from build123d import *

# Parameters (mm, degrees)
SKETCH_1_R          = 25.5
EXTRUDE_1_DEPTH     = 13
SKETCH_2_R          = 23.5
CUT_EXTRUDE_1_DEPTH = 11
SKETCH_3_R          = 22
CUT_EXTRUDE_2_DEPTH = 2
EXTRUDE_START       = -3
SKETCH_4_R          = 35.5
SKETCH_4_R_2        = 25.5
EXTRUDE_2_DEPTH     = 3
SKETCH_5_R          = 1.575
CUT_EXTRUDE_3_DEPTH = 52.860389509


with BuildPart() as part:
    # 草图1 → 凸台-拉伸1 (new body)
    with BuildSketch(Plane.XY):
        with Locations(Location((0, 0, 0), (0, 0, 180))):
            Circle(SKETCH_1_R)
    extrude(amount=EXTRUDE_1_DEPTH)

    # 草图2 → 切除-拉伸1 (cut)
    with BuildSketch(Plane(origin=(0, 0, 0), x_dir=(-1, 0, 0), z_dir=(0, 0, -1))):
        Circle(SKETCH_2_R)
    extrude(amount=-CUT_EXTRUDE_1_DEPTH, mode=Mode.SUBTRACT)

    # 草图3 → 切除-拉伸2 (cut)
    with BuildSketch(Plane.XY.offset(13)):
        Circle(SKETCH_3_R)
    extrude(amount=-CUT_EXTRUDE_2_DEPTH, mode=Mode.SUBTRACT)

    # 草图4 → 凸台-拉伸2 (add)
    with BuildSketch(Plane.XY.offset(13).offset(EXTRUDE_START)):
        Circle(SKETCH_4_R)
        with Locations(Location((0, 0, 0), (0, 0, 180))):
            Circle(SKETCH_4_R_2, mode=Mode.SUBTRACT)
    extrude(amount=EXTRUDE_2_DEPTH)

    # 草图5 → 切除-拉伸3 (cut, through all)
    with BuildSketch(Plane.XY.offset(13)):
        with Locations((0, 30.5)):
            Circle(SKETCH_5_R)
        with Locations((30.5, 0)):
            Circle(SKETCH_5_R)
        with Locations((0, -30.5)):
            Circle(SKETCH_5_R)
        with Locations((-30.5, 0)):
            Circle(SKETCH_5_R)
    extrude(amount=-CUT_EXTRUDE_3_DEPTH, mode=Mode.SUBTRACT)


solid = part.part
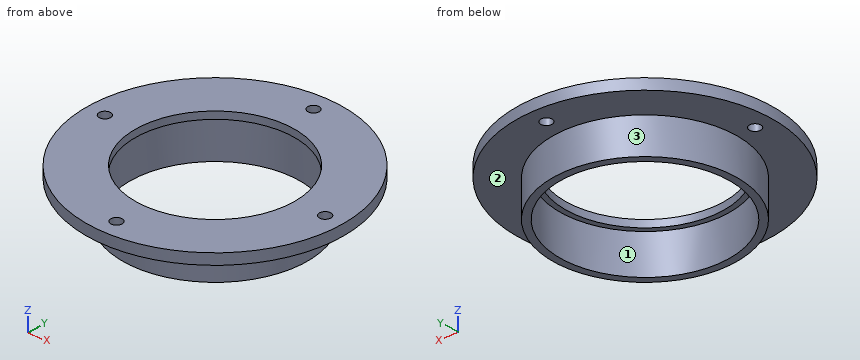
Work out the finished part from the listing and answer in its coordinate system (mm). Face numbers are marked on the shaded views. Round coordinates to 2 decimals unless told otherwise and drop trailing zeros. Write each loop counter-clockwise with the first axis right and the second up, starting at its lowest first coordinate (ties: lowest second). Pieces come first, ordered by that corner, then holes. Notation, with made-up numbers: (31.5, 49.25) - (45.5, 49.25) arc R18 cw to (45.5, 71.25) - close; hole circle Ø10 at (-20, 37.5). An arc over 180 degrees is marked (long way). Answer in a Markdown table with one row per item. Add a question column.
1. Given pin 1 (5 mm diameter, centred on x = 0, y = -30.5, fed in from +Z); pin 2 (1.9 mm diameter, centred on x = 30.5, y = 0, fed in from -Z); pin 3 (5 mm diameter, centred on x = -5.5, z = 7, fed in from +Y); pin 4 (3 mm diameter, centred on x = -2.5, z = 10, fed in from -Y), each flat-ended and moving along its own axis, determine where each tip first touches the part or whether it passes through.
2. Find the intervals of material crossed by line 1 along Y through (x, z) = (0, 11.55) (3 decimals); line 2 along Y through (x, z) = (0, 10.75) (3 decimals); line 3 along Z through (x, y) = (18.5, -19), in increasing order. Write a range as from..to.
3. A cutting plane is placed at A-A, the plane y = 0. Determine the outline of the cut face in (x, z) (3 decimals), and give its area (3 significant figures).
4. A cutting plane is placed at D-D, the plane x = 30.5. Determine the outline of the cut face in (y, z) (3 decimals).
5. The mould has two halves that part along Y. Classify the marked faces 1, 2 and 3: +Y half, -Y half, draft (parallel to the pull), parting line (faces both ways), or undercut.
6. A cutting plane is placed at C-C, the plane y = -15. Determine the outline of the cut face in (x, z), and give its area (3 significant figures).
Worked out:
| question | item | result |
|---|---|---|
| 1 | pin 1 | z = 13 |
| 1 | pin 2 | through |
| 1 | pin 3 | y = 25.32 |
| 1 | pin 4 | y = -35.49 |
| 2 | line 1 | -35.5..-32.075, -28.925..-22, 22..28.925, 32.075..35.5 |
| 2 | line 2 | -35.5..-32.075, -28.925..-23.5, 23.5..28.925, 32.075..35.5 |
| 2 | line 3 | 10..13 |
| 3 | outline | (-35.5, 10) - (-32.075, 10) - (-32.075, 13) - (-35.5, 13) - close; (-28.925, 10) - (-25.5, 10) - (-25.5, 0) - (-23.5, 0) - (-23.5, 11) - (-22, 11) - (-22, 13) - (-28.925, 13) - close; (22, 11) - (23.5, 11) - (23.5, 0) - (25.5, 0) - (25.5, 10) - (28.925, 10) - (28.925, 13) - (22, 13) - close; (32.075, 10) - (35.5, 10) - (35.5, 13) - (32.075, 13) - close |
| 3 | area | 99.1 mm^2 |
| 4 | outline | (-18.166, 10) - (-1.575, 10) - (-1.575, 13) - (-18.166, 13) - close; (1.575, 10) - (18.166, 10) - (18.166, 13) - (1.575, 13) - close |
| 5 | face 1 | undercut |
| 5 | face 2 | draft |
| 5 | face 3 | parting line |
| 6 | outline | (-32.18, 10) - (-20.62, 10) - (-20.62, 0) - (-18.09, 0) - (-18.09, 11) - (-16.09, 11) - (-16.09, 13) - (-32.18, 13) - close; (16.09, 11) - (18.09, 11) - (18.09, 0) - (20.62, 0) - (20.62, 10) - (32.18, 10) - (32.18, 13) - (16.09, 13) - close |
| 6 | area | 143 mm^2 |
